For this review, take the finished solid that the model builds, in its own axes (mm). Face numbers are marked on the shaded views. Give positions to 0.01 mm unless a question says otherwise; leave off trailing zeros. Write each loop counter-clockwise with the first axis right and the second up, starting at its lowest first coordinate (ties: lowest second). Pieces come first, ordered by that corner, then holes. Notation, with made-up numbers: (-11.5, -11) -> (15.5, -11) arc R22 ccw to (15.5, 4) -> close; hole circle Ø7 at (77, 2.25). An arc over 180 degrees is marked (long way). Write item = value, one per line.
```python
from build123d import *

# Parameters (mm, degrees)
SKETCH1_W           = 38.1
SKETCH1_H           = 21.209
BOSS_EXTRUDE1_DEPTH = 6.35
SKETCH2_R           = 2.667
CUT_EXTRUDE1_DEPTH  = 9.525
CUT_EXTRUDE2_DEPTH  = 9.525


with BuildPart() as part:
    # Sketch1 → Boss-Extrude1 (new body)
    with BuildSketch(Plane(origin=(0, 0, 0), x_dir=(1, 0, 0), z_dir=(0, 1, 0))):
        Rectangle(SKETCH1_W, SKETCH1_H)
    extrude(amount=BOSS_EXTRUDE1_DEPTH)

    # Sketch2 → Cut-Extrude1 (cut)
    with BuildSketch(Plane(origin=(0, 6.35, 0), x_dir=(1, 0, 0), z_dir=(0, 1, 0))):
        with Locations((-12.7, 0)):
            Circle(SKETCH2_R)
        with Locations((12.7, 0)):
            Circle(SKETCH2_R)
    extrude(amount=-CUT_EXTRUDE1_DEPTH, mode=Mode.SUBTRACT)

    # Sketch3 → Cut-Extrude2 (cut)
    with BuildSketch(Plane(origin=(0, 6.35, 0), x_dir=(1, 0, 0), z_dir=(0, 1, 0))):
        Polygon((-19.05, 10.6045), (-15.875, 10.6045), (-19.05, 7.4295), align=None)
        Polygon((19.05, 10.6045), (15.748, 10.6045), (19.05, 7.3025), align=None)
        Polygon((19.05, -10.6045), (15.748, -10.6045), (19.05, -7.3025), align=None)
        Polygon((-19.05, -10.6045), (-15.875, -10.6045), (-19.05, -7.4295), align=None)
    extrude(amount=-CUT_EXTRUDE2_DEPTH, mode=Mode.SUBTRACT)


solid = part.part
```
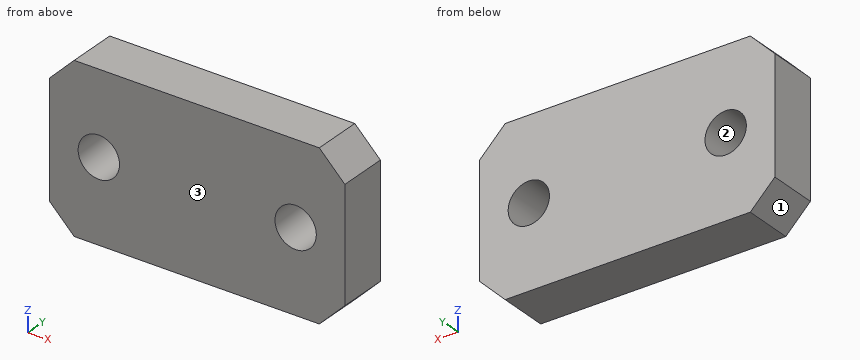
(1) The part is to be moulded in two halves that separate along X. For the marked faces 1, 2 and 3, say which applies: released by +X, released by -X, zero draft, split by the parting line, or undercut.
Answers below:
face_1 = released by -X
face_2 = undercut
face_3 = zero draft
(2) Take a section at C-C (y = 4.25). Count the separate pieces of the cut face and the enclosed holes in it, plus the area to 3 significant figures.
Answers below:
separate_pieces = 1
enclosed_holes = 2
area = 742 mm^2
(3) Take a section at B-B (z = 0). Write out the cut boundary in (x, y).
Answers below:
outline = (-19.05, 0) -> (-15.37, 0) -> (-15.37, 6.35) -> (-19.05, 6.35) -> close; (-10.03, 0) -> (10.03, 0) -> (10.03, 6.35) -> (-10.03, 6.35) -> close; (15.37, 0) -> (19.05, 0) -> (19.05, 6.35) -> (15.37, 6.35) -> close
(4) Take a section at D-D (z = -8). Write out the cut boundary in (x, y).
Answers below:
outline = (-18.48, 0) -> (18.35, 0) -> (18.35, 6.35) -> (-18.48, 6.35) -> close
(5) Take a section at A-A (x = -12.7). Write out the cut boundary in (y, z).
Answers below:
outline = (0, -10.6) -> (6.35, -10.6) -> (6.35, -2.67) -> (0, -2.67) -> close; (0, 2.67) -> (6.35, 2.67) -> (6.35, 10.6) -> (0, 10.6) -> close
(6) To check wall thickness, follow probe 1 along X at (y, z) = (2, 0); probe 2 along Z at (x, y) = (-12.5, 3.25); probe 3 along X at (y, z) = (5.75, 2). State the ranges of each line that lie inside material, in increasing order.
Answers below:
probe_1 = -19.05 to -15.37, -10.03 to 10.03, 15.37 to 19.05
probe_2 = -10.6 to -2.66, 2.66 to 10.6
probe_3 = -19.05 to -14.46, -10.94 to 10.94, 14.46 to 19.05
